Answer from the drawing. Dimensions are ordinates in mm from the lowest x, y and z of the part. Coordinates: 2 decimals unless noted, no trailing zeros. Write each loop counter-clockwise with the first axis right and the second up, starting at its lowest first coordinate (ties: lowest second). Pieces come first, ordered by that corner, then holes. Notation, with made-up numbers: (69, 13) - (114, 13) arc R13 ccw to (114, 27) - close; hole circle Ø3 at (-29.75, 86). An arc over 180 degrees is marked (long way). Use a Markdown table: item, result.
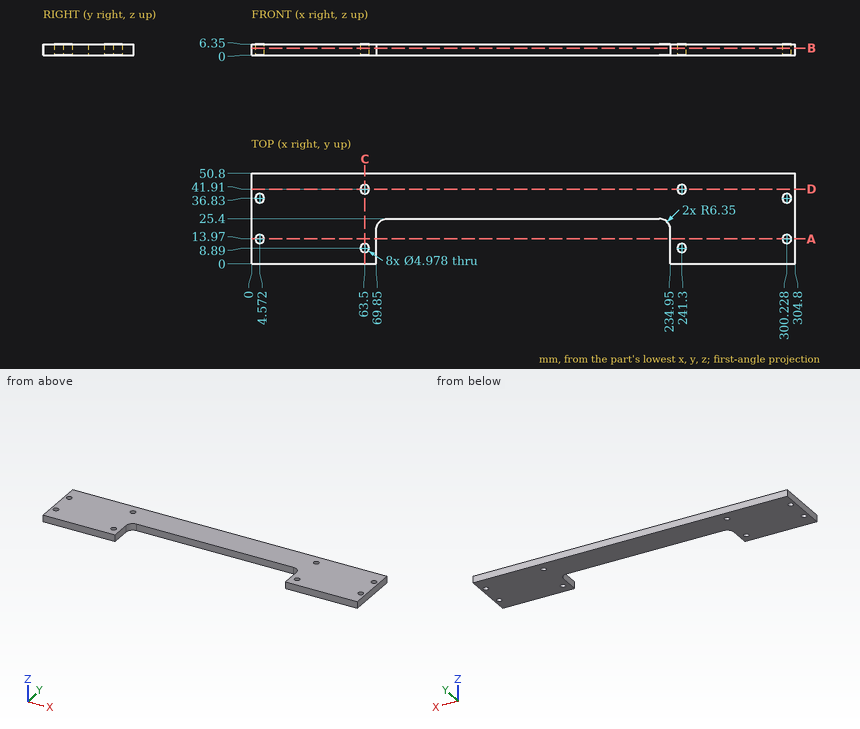
(1) A cutting plane is placed at D-D, the plane y = 41.91. Write down the section's boundary in (x, z).
Report:
| item | result |
|---|---|
| outline | (0, 0) - (61.01, 0) - (61.01, 6.35) - (0, 6.35) - close; (65.99, 0) - (238.81, 0) - (238.81, 6.35) - (65.99, 6.35) - close; (243.79, 0) - (304.8, 0) - (304.8, 6.35) - (243.79, 6.35) - close |
(2) A cutting plane is placed at B-B, the plane z = 4. Count the separate pieces of the cut face and the enclosed holes in it, and give its area (3 significant figures).
Report:
| item | result |
|---|---|
| separate pieces | 1 |
| enclosed holes | 8 |
| area | 11,200 mm² |
(3) A cutting plane is placed at A-A, the plane y = 13.97. Write down the section's boundary in (x, z), and give its area (3 significant figures).
Report:
| item | result |
|---|---|
| outline | (0, 0) - (2.08, 0) - (2.08, 6.35) - (0, 6.35) - close; (7.06, 0) - (69.85, 0) - (69.85, 6.35) - (7.06, 6.35) - close; (234.95, 0) - (297.74, 0) - (297.74, 6.35) - (234.95, 6.35) - close; (302.72, 0) - (304.8, 0) - (304.8, 6.35) - (302.72, 6.35) - close |
| area | 824 mm² |
(4) A cutting plane is placed at C-C, the plane x = 63.5. Write down the section's boundary in (y, z).
Report:
| item | result |
|---|---|
| outline | (0, 0) - (6.4, 0) - (6.4, 6.35) - (0, 6.35) - close; (11.38, 0) - (39.42, 0) - (39.42, 6.35) - (11.38, 6.35) - close; (44.4, 0) - (50.8, 0) - (50.8, 6.35) - (44.4, 6.35) - close |
(5) Straight lines are drawn through the part: L1, parallel to Y at x = 241.3, z = 5; L2, parallel to X at y = 5, z = 2; L3, parallel to Y at x = 107.5, z = 5.5. For each, find the intervals that lie inside material, in ascending order.
Report:
| item | result |
|---|---|
| L1 | y = 0 to 6.4, 11.38 to 39.42, 44.4 to 50.8 |
| L2 | x = 0 to 69.85, 234.95 to 304.8 |
| L3 | y = 25.4 to 50.8 |
(6) Each of these flat-tipped pins is pushed along its axis until it touches: P1, Ø3, axis at x = 83.5, z = 5.5, coming from the -Y side; P2, Ø4, axis at x = 63.5, y = 41.91, coming from the +Z side; P3, Ø3, axis at x = 249, y = 16, coming from the -Z side. Where does it stop, or does it pass through?
Report:
| item | result |
|---|---|
| P1 | stops at y = 25.4 |
| P2 | passes through |
| P3 | stops at z = 0 |
